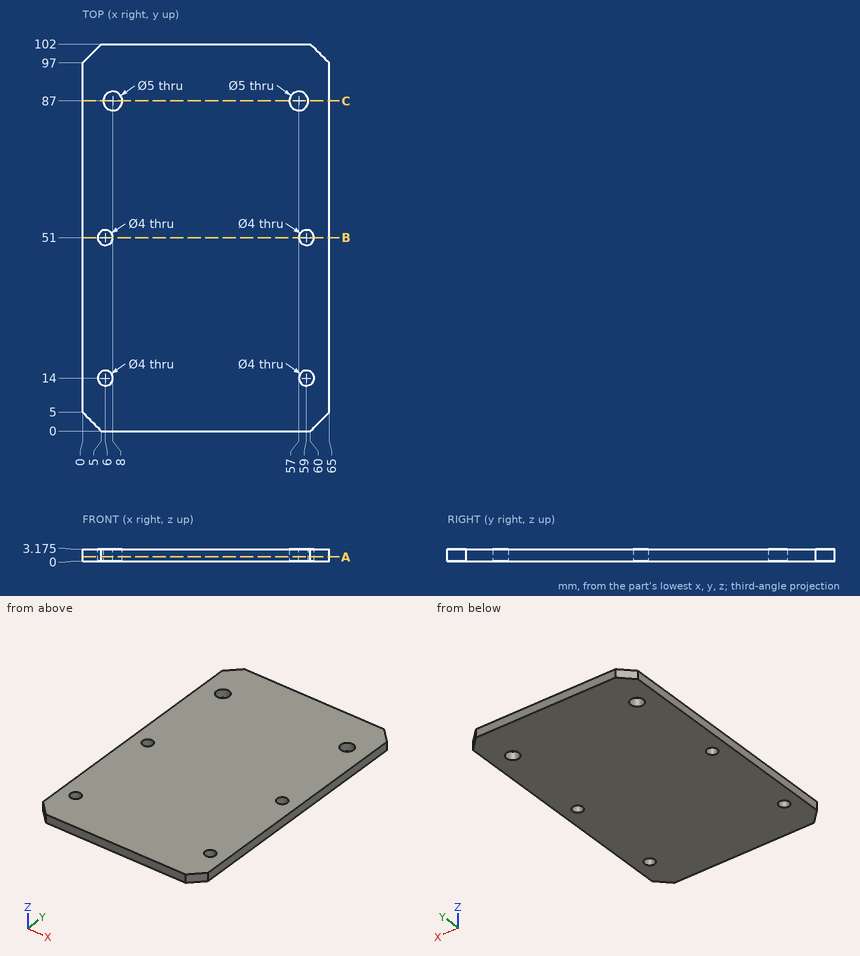
Study the drawing (mm; zero at the part's minimum x, y, z) and answer. Give positions to 0.01 mm unless a question says otherwise; leave off trailing zeros. Order: outer loops, then holes, each group sorted by start corner. A loop starts at its lowest first (then second) coordinate and runs counter-clockwise, first axis right, second up. Notation, with made-up numbers: (61.5, 61.5) -> (80.5, 61.5) arc R16 cw to (80.5, 70.5) -> close; hole circle Ø9 at (-21, 36). An arc over 180 degrees is marked (long way). Put each result on its own line as item: value.
Item 1: Given P1, Ø2.5, axis at x = 6, y = 51, coming from the -Z side, flat-ended and moving along its own axis, determine where the tip first touches the part or whether it passes through.
Established:
P1: passes through
Item 2: A cutting plane is placed at B-B on y = 51. Give the vertices of the cut face in (x, z) (3 decimals), plus the area to 3 significant figures.
Established:
outline: (0, 0) -> (4, 0) -> (4, 3.175) -> (0, 3.175) -> close; (8, 0) -> (57, 0) -> (57, 3.175) -> (8, 3.175) -> close; (61, 0) -> (65, 0) -> (65, 3.175) -> (61, 3.175) -> close
area: 181 mm^2
Item 3: A cutting plane is placed at A-A on z = 1.15. Give the vertices of the cut face in (x, y), plus the area to 3 significant figures.
Established:
outline: (0, 5) -> (5, 0) -> (60, 0) -> (65, 5) -> (65, 97) -> (60, 102) -> (5, 102) -> (0, 97) -> close; hole circle Ø4 at (6, 14); hole circle Ø4 at (6, 51); hole circle Ø5 at (8, 87); hole circle Ø5 at (57, 87); hole circle Ø4 at (59, 14); hole circle Ø4 at (59, 51)
area: 6,490 mm^2
Item 4: Straight lines are drawn through the part: line 1 (X direction, y = 87, z = 1.35); line 2 (Y direction, x = 59, z = 0.7); line 3 (X direction, y = 85.5, z = 2.1). For each, find the intervals that lie inside material, in ascending order.
Established:
line 1: x = 0 to 5.5, 10.5 to 54.5, 59.5 to 65
line 2: y = 0 to 12, 16 to 49, 53 to 85.5, 88.5 to 102
line 3: x = 0 to 6, 10 to 55, 59 to 65
Item 5: A cutting plane is placed at C-C on y = 87. Give the vertices of the cut face in (x, z) (3 decimals), plus the area to 3 significant figures.
Established:
outline: (0, 0) -> (5.5, 0) -> (5.5, 3.175) -> (0, 3.175) -> close; (10.5, 0) -> (54.5, 0) -> (54.5, 3.175) -> (10.5, 3.175) -> close; (59.5, 0) -> (65, 0) -> (65, 3.175) -> (59.5, 3.175) -> close
area: 175 mm^2
